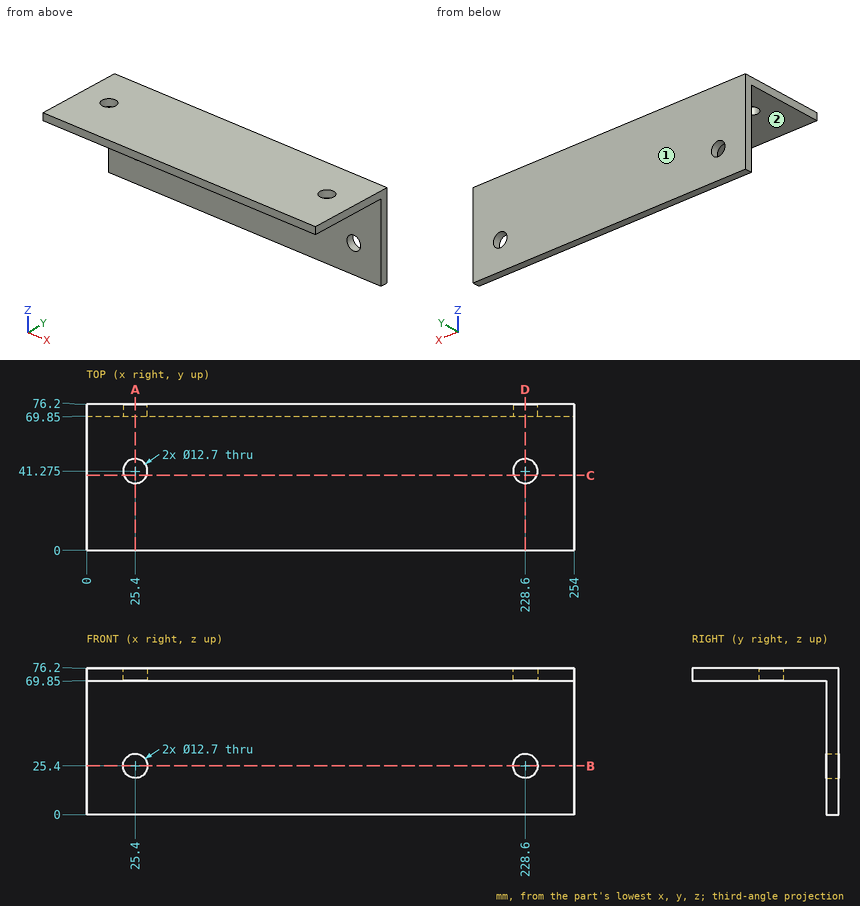
Check sheet for the drawn part. Datum: minimum x, y, z corner. Units: mm. A direction names the side the tool comes from. Round coordinates to 2 decimals unless told otherwise and drop trailing zeros. Order: outer loops, then holes, each group sorted by start corner. A loop starts at its lowest first (then second) coordinate and runs counter-clockwise, first axis right, second up. Notation, with made-up numbers: M 0,-21 L 39,-21 A27 cw 39,16 Z; hole C 86,-29 d9. An arc over 180 degrees is marked long. Answer in a Markdown table with one row per item.
(1) Gauge pin test, flat ends, axial feed: pin 1 (10 mm diameter, centred on x = 158.5, z = 25, fed in from -Y); pin 2 (3 mm diameter, centred on x = 40.5, y = 11.5, fed in from -Z). Record the tip position at first contact, or that the pin passes through.
Findings:
| item | result |
|---|---|
| pin 1 | stops at y = 69.85 |
| pin 2 | stops at z = 69.85 |
(2) Set-up check for the marked faces 1 and 2: record each of +Z, -Z, +X, -X, +Y, -Y from which the full face is reachable in a straight line by a thin tool's end or side.
Findings:
| item | result |
|---|---|
| face 1 | +Z, -Z, +X, -X, +Y |
| face 2 | -Z, +X, -X, -Y |
(3) Section check B-B on z = 25.4. Record the boundary of the cut face in (x, y).
Findings:
| item | result |
|---|---|
| outline | M 0,69.85 L 19.05,69.85 L 19.05,76.2 L 0,76.2 Z; M 31.75,69.85 L 222.25,69.85 L 222.25,76.2 L 31.75,76.2 Z; M 234.95,69.85 L 254,69.85 L 254,76.2 L 234.95,76.2 Z |
(4) Section check C-C on y = 39. Record the boundary of the cut face in (x, z).
Findings:
| item | result |
|---|---|
| outline | M 0,69.85 L 19.47,69.85 L 19.47,76.2 L 0,76.2 Z; M 31.33,69.85 L 222.67,69.85 L 222.67,76.2 L 31.33,76.2 Z; M 234.53,69.85 L 254,69.85 L 254,76.2 L 234.53,76.2 Z |
(5) Section check D-D on x = 228.5. Record the boundary of the cut face in (y, z).
Findings:
| item | result |
|---|---|
| outline | M 0,69.85 L 34.93,69.85 L 34.93,76.2 L 0,76.2 Z; M 47.62,69.85 L 69.85,69.85 L 69.85,31.75 L 76.2,31.75 L 76.2,76.2 L 47.62,76.2 Z; M 69.85,0 L 76.2,0 L 76.2,19.05 L 69.85,19.05 Z |
(6) Material ranges on line 1 along X through (y, z) = (72, 25); line 2 along Y through (x, z) = (228, 72); line 3 along Z through (x, y) = (25.4, 74.5), recorded low to high. Write a range as from..to.
Findings:
| item | result |
|---|---|
| line 1 | x = 0..19.06, 31.74..222.26, 234.94..254 |
| line 2 | y = 0..34.95, 47.6..76.2 |
| line 3 | z = 0..19.05, 31.75..76.2 |
(7) Section check A-A on x = 25.4. Record the boundary of the cut face in (y, z) (3 decimals).
Findings:
| item | result |
|---|---|
| outline | M 0,69.85 L 34.925,69.85 L 34.925,76.2 L 0,76.2 Z; M 47.625,69.85 L 69.85,69.85 L 69.85,31.75 L 76.2,31.75 L 76.2,76.2 L 47.625,76.2 Z; M 69.85,0 L 76.2,0 L 76.2,19.05 L 69.85,19.05 Z |
